from build123d import *

# Parameters (mm, degrees)
SKETCH1_W           = 20
SKETCH1_H           = 3
BOSS_EXTRUDE1_DEPTH = 3


with BuildPart() as part:
    # Sketch1 → Boss-Extrude1 (new body)
    # profile 1 of 3: a face of its own
    with BuildSketch(Plane.XY):
        Polygon((35, 40), (-35, 40), (-38, 40), (-38, 37.5), (-35, 37.5), (-35, 22.5), (-38, 22.5), (-38, 7.5), (-35, 7.5), (-35, -7.5), (-38, -7.5), (-38, -22.5), (-35, -22.5), (-35, -37.5), (-38, -37.5), (-38, -40), (-27.5, -40), (-7.5, -40), (7.5, -40), (27.5, -40), (38, -40), (38, -37.5), (35, -37.5), (35, -22.5), (38, -22.5), (38, -7.5), (35, -7.5), (35, 7.5), (38, 7.5), (38, 22.5), (35, 22.5), (35, 37.5), (38, 37.5), (38, 40), align=None)
        with BuildLine():
            Line((-15, 27.5), (-15, -27.5))
            ThreePointArc((-15, -27.5), (-20, -32.5), (-25, -27.5))
            Line((-25, -27.5), (-25, 27.5))
            ThreePointArc((-25, 27.5), (-20, 32.5), (-15, 27.5))
        make_face(mode=Mode.SUBTRACT)
        with BuildLine():
            ThreePointArc((5, -27.5), (0, -32.5), (-5, -27.5))
            Line((-5, -27.5), (-5, 27.5))
            ThreePointArc((-5, 27.5), (0, 32.5), (5, 27.5))
            Line((5, 27.5), (5, -27.5))
        make_face(mode=Mode.SUBTRACT)
        with BuildLine():
            ThreePointArc((25, -27.5), (20, -32.5), (15, -27.5))
            Line((15, -27.5), (15, 27.5))
            ThreePointArc((15, 27.5), (20, 32.5), (25, 27.5))
            Line((25, 27.5), (25, -27.5))
        make_face(mode=Mode.SUBTRACT)
    # profile 2 of 3: a face of its own
    with BuildSketch(Plane.XY):
        with Locations((17.5, -41.5)):
            Rectangle(SKETCH1_W, SKETCH1_H)
    # profile 3 of 3: a face of its own
    with BuildSketch(Plane.XY):
        with Locations((-17.5, -41.5)):
            Rectangle(SKETCH1_W, SKETCH1_H)
    extrude(amount=BOSS_EXTRUDE1_DEPTH)


solid = part.part
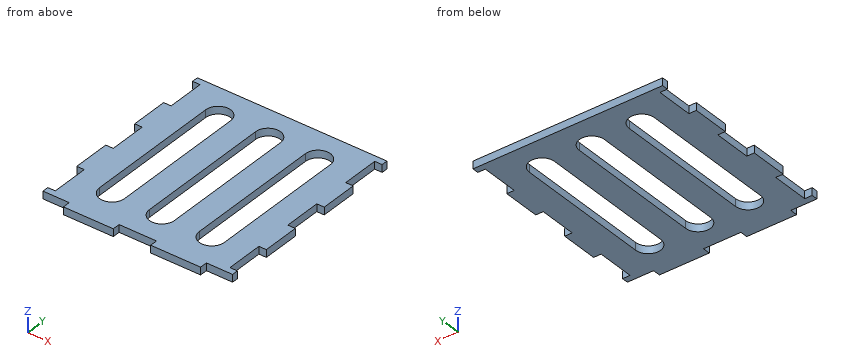
Work out the finished part from the listing and answer in its coordinate system (mm). Give positions to 0.01 mm unless a question says otherwise; leave off trailing zeros. Loops run counter-clockwise (first coordinate to the right, second up) from the corner with the lowest first, then second, coordinate; pieces in that order, holes last. Notation, with made-up numbers: (-24, 28) - (13, 28) arc R24 ccw to (13, 42) - close; hole circle Ø10 at (30.5, 60). An arc over 180 degrees is marked (long way). Answer in a Markdown table with one row per item.
(1) Consider L1, parallel to X at y = 20.5, z = 2.35; L2, parallel to X at y = -3, z = 1.15; L3, parallel to Y at x = -32, z = 0.95. Determine where each line is inside the solid, lowest interval first. Write a range as [from, to].
Results list:
| item | result |
|---|---|
| L1 | x = [-38, -25], [-15, -5], [5, 15], [25, 38] |
| L2 | x = [-35, -25], [-15, -5], [5, 15], [25, 35] |
| L3 | y = [-40, 40] |
(2) Section B-B (y = 25) is taken. Give the vertices of the cut face in (x, z).
Results list:
| item | result |
|---|---|
| outline | (-35, 0) - (-25, 0) - (-25, 3) - (-35, 3) - close; (-15, 0) - (-5, 0) - (-5, 3) - (-15, 3) - close; (5, 0) - (15, 0) - (15, 3) - (5, 3) - close; (25, 0) - (35, 0) - (35, 3) - (25, 3) - close |
(3) Flat-ended cylindrical pins translate along their axes: pin 1 Ø1.5 at (y, z) = (-27, 1.5) entering from +X; pin 2 Ø1.5 at (y, z) = (-41, 1.5) entering from -X; pin 3 Ø0.9 at (x, z) = (37, 1.5) entering from -Y. Find the tip coordinate at first contact, or state that the pin passes through.
Results list:
| item | result |
|---|---|
| pin 1 | stops at x = 35 |
| pin 2 | stops at x = -27.5 |
| pin 3 | stops at y = -40 |
(4) Section D-D (z = 1.75) is taken. State how many separate pieces and enclosed holes the cut face has, and give its area (3 significant figures).
Results list:
| item | result |
|---|---|
| separate pieces | 1 |
| enclosed holes | 3 |
| area | 4,040 mm² |
(5) Section C-C (y = 15.5) is taken. Give the vertices of the cut face in (x, z), and give its area (3 significant figures).
Results list:
| item | result |
|---|---|
| outline | (-38, 0) - (-25, 0) - (-25, 3) - (-38, 3) - close; (-15, 0) - (-5, 0) - (-5, 3) - (-15, 3) - close; (5, 0) - (15, 0) - (15, 3) - (5, 3) - close; (25, 0) - (38, 0) - (38, 3) - (25, 3) - close |
| area | 138 mm² |
(6) Section A-A (x = 16) is taken. Give the vertices of the cut face in (y, z).
Results list:
| item | result |
|---|---|
| outline | (-43, 0) - (-30.5, 0) - (-30.5, 3) - (-43, 3) - close; (30.5, 0) - (40, 0) - (40, 3) - (30.5, 3) - close |
